Geometry: final body of the model. Coordinates: model frame, mm. Coordinates: 2 decimals unless noted, no trailing zeros. Loops run counter-clockwise (first coordinate to the right, second up) from the corner with the lowest first, then second, coordinate; pieces in that order, holes last. Notation, with made-up numbers: (56, 35) - (108, 35) arc R26 cw to (108, 70) - close; hole circle Ø1 at (23.5, 43.25). An arc over 180 degrees is marked (long way). Put each result on its own line as item: value. Start each with the question number.
1) Material intervals for line 1 along X through (y, z) = (650, 1.95); line 2 along X through (y, z) = (131, 7.5); line 3 along Z through (x, y) = (-23.5, 371), sorted ascending. Write a range as from..to.
2) Contact query for flat-ended pins moving along their axis: pin 1 Ø6 at (x, y) = (17.5, 1250) entering from -Z; pin 2 Ø1.5 at (y, z) = (638, 33) entering from +X; pin 3 Ø7.5 at (x, y) = (-17.5, 250) entering from +Z; pin 4 Ø8 at (y, z) = (836, 33) entering from -X. Output: stop coordinate, or through.
3) Section A-A on y = 958.5. Output: boundary loops of the cut face in (x, z), and give its area (3 significant figures).
4) Section B-B on z = 30. Output: boundary loops of the cut face in (x, y), and give its area (3 significant figures).
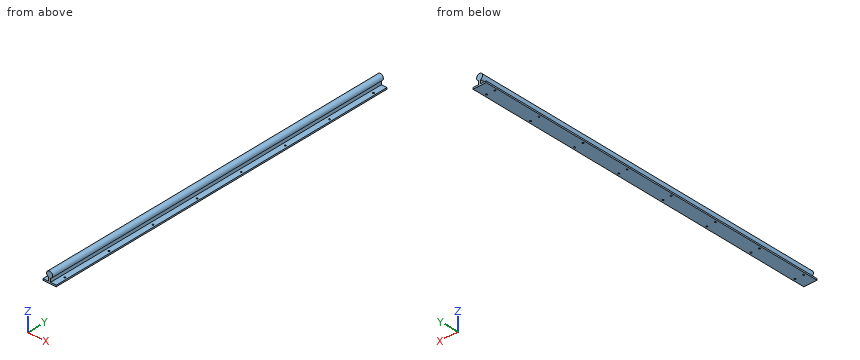
```python
from build123d import *

# Parameters (mm, degrees)
F2_DEPTH = 1500
F1_R     = 3.3
F3_DEPTH = 3


with BuildPart() as f2:
    # F0 (on Front) → F2 (new body)
    with BuildSketch(Plane.XZ):
        with BuildLine():
            Line((27.5, -3), (27.5, 3))
            Line((27.5, 3), (4, 3))
            Line((4, 3), (4, 18.1572807177))
            ThreePointArc((4, 18.1572807177), (0, 42.5), (-4, 18.1572807177))
            Line((-4, 18.1572807177), (-4, 3))
            Line((-4, 3), (-27.5, 3))
            Line((-27.5, 3), (-27.5, -3))
            Line((-27.5, -3), (27.5, -3))
        make_face()
    extrude(amount=-F2_DEPTH)

    # F1 (on Top) → F3 (cut, symmetric)
    with BuildSketch(Plane.XY):
        with Locations((17.5, 50)):
            Circle(F1_R)
        with Locations((17.5, 250)):
            Circle(F1_R)
        with Locations((17.5, 1050)):
            Circle(F1_R)
        with Locations((17.5, 450)):
            Circle(F1_R)
        with Locations((17.5, 650)):
            Circle(F1_R)
        with Locations((17.5, 850)):
            Circle(F1_R)
        with Locations((17.5, 1250)):
            Circle(F1_R)
        with Locations((17.5, 1450)):
            Circle(F1_R)
        with Locations((-17.5, 50)):
            Circle(F1_R)
        with Locations((-17.5, 250)):
            Circle(F1_R)
        with Locations((-17.5, 450)):
            Circle(F1_R)
        with Locations((-17.5, 650)):
            Circle(F1_R)
        with Locations((-17.5, 850)):
            Circle(F1_R)
        with Locations((-17.5, 1450)):
            Circle(F1_R)
        with Locations((-17.5, 1250)):
            Circle(F1_R)
        with Locations((-17.5, 1050)):
            Circle(F1_R)
    extrude(amount=F3_DEPTH, both=True, mode=Mode.SUBTRACT)


solid = f2.part
```
Answer block:
1. line 1: x = -27.5..-20.8, -14.2..14.2, 20.8..27.5
1. line 2: x = -4..4
1. line 3: z = -3..3
2. pin 1: passes through
2. pin 2: stops at x = 12.3
2. pin 3: stops at z = 3
2. pin 4: stops at x = -12.5
3. outline: (-27.5, -3) - (27.5, -3) - (27.5, 3) - (4, 3) - (4, 18.16) arc R12.5 ccw (long way) to (-4, 18.16) - (-4, 3) - (-27.5, 3) - close
3. area: 939 mm²
4. outline: (-12.5, 0) - (12.5, 0) - (12.5, 1500) - (-12.5, 1500) - close
4. area: 37,500 mm²
